Design review of the part built by this model. Coordinates are the model's own, in mm. Face numbers are marked on the shaded views. Give positions to 0.01 mm unless a question says otherwise; leave off trailing zeros. Loops run counter-clockwise (first coordinate to the right, second up) from the corner with the lowest first, then second, coordinate; pieces in that order, holes last.
from build123d import *

# Parameters (mm, degrees)
SKETCH1_R           = 6.5
BOSS_EXTRUDE1_DEPTH = 4
SKETCH2_R           = 2.75
CUT_EXTRUDE1_DEPTH  = 7
SKETCH3_R           = 0.9
CUT_EXTRUDE2_DEPTH  = 7


with BuildPart() as part:
    # Sketch1 → Boss-Extrude1 (new body)
    with BuildSketch(Plane(origin=(0, 0, 0), x_dir=(0, 0, -1), z_dir=(1, 0, 0))):
        Circle(SKETCH1_R)
    extrude(amount=BOSS_EXTRUDE1_DEPTH)

    # Sketch2 → Cut-Extrude1 (cut)
    with BuildSketch(Plane(origin=(4, 0, 0), x_dir=(0, 0, -1), z_dir=(1, 0, 0))):
        Circle(SKETCH2_R)
    extrude(amount=-CUT_EXTRUDE1_DEPTH, mode=Mode.SUBTRACT)

    # Sketch3 → Cut-Extrude2 (cut)
    with BuildSketch(Plane.ZY):
        with Locations((-2.001020721, 3.230466851)):
            Circle(SKETCH3_R)
        with Locations((3.798176719, 0.117701352)):
            Circle(SKETCH3_R)
        with Locations((-1.797155999, -3.348168203)):
            Circle(SKETCH3_R)
    extrude(amount=-CUT_EXTRUDE2_DEPTH, mode=Mode.SUBTRACT)


solid = part.part
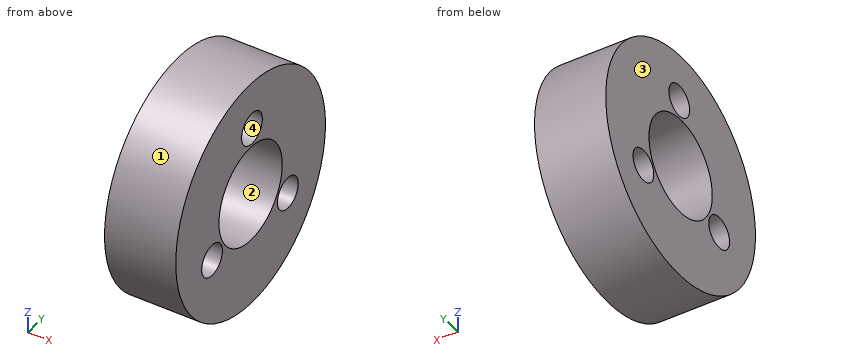
Q1. Take a section at B-B (y = 2.5). Give the boundary of the cut face in (x, z), plus the area to 3 significant figures.
Results:
outline: (0, -6) - (4, -6) - (4, -2.53) - (0, -2.53) - close; (0, -1.48) - (4, -1.48) - (4, -1.15) - (0, -1.15) - close; (0, 1.15) - (4, 1.15) - (4, 6) - (0, 6) - close
area: 34.6 mm2
Q2. Take a section at D-D (x = 0.4). Give the boundary of the cut face in (y, z).
Results:
outline: circle Ø13 at (0, 0); hole circle Ø1.8 at (-3.35, -1.8); hole circle Ø5.5 at (0, 0); hole circle Ø1.8 at (0.12, 3.8); hole circle Ø1.8 at (3.23, -2)
Q3. Take a section at C-C (z = -1.75). Give the boundary of the cut face in (x, y), plus the area to 3 significant figures.
Results:
outline: (0, -6.26) - (4, -6.26) - (4, -4.25) - (0, -4.25) - close; (0, -2.45) - (4, -2.45) - (4, -2.12) - (0, -2.12) - close; (0, 2.12) - (4, 2.12) - (4, 2.37) - (0, 2.37) - close; (0, 4.09) - (4, 4.09) - (4, 6.26) - (0, 6.26) - close
area: 19.0 mm2
Q4. Take a section at A-A (z = 0). Give the boundary of the cut face in (x, y).
Results:
outline: (0, -6.5) - (4, -6.5) - (4, -2.75) - (0, -2.75) - close; (0, 2.75) - (4, 2.75) - (4, 6.5) - (0, 6.5) - close
Q5. Wall thickness on line 1 (Z direction, x = 3.4, y = 2.5); line 2 (Z direction, x = 1, y = -0.5); line 3 (Y direction, x = 0.4, z = -2.25): over which ranges is each line inside the solid? List them lowest first.
Results:
line 1: z = -6 to -2.53, -1.48 to -1.15, 1.15 to 6
line 2: z = -6.48 to -2.7, 2.7 to 3.14, 4.45 to 6.48
line 3: y = -6.1 to -4.13, -2.57 to -1.58, 1.58 to 2.37, 4.1 to 6.1
Q6. Insertion check: pin 1 (1 mm diameter, centred on x = 3, z = -1.5, fed in from -Y); pin 2 (1.5 mm diameter, centred on x = 1.5, y = 1, fed in from -Z); pin 3 (1 mm diameter, centred on x = 2.5, y = 3, fed in from -Z). Each pin has a flat end and moves straight along its axis. Give the tip position at first contact, or say it passes through.
Results:
pin 1: stops at y = -6.42
pin 2: stops at z = -6.5
pin 3: stops at z = -6
Q7. Draft analysis for pull direction Y (two halves, no side actions). For the marked faces 1, 2, 3 and 4, state which applies: pulls with the +Y half, pulls with the -Y half, needs draft (parallel to the pull), parting line crosses it, or undercut.
Results:
face 1: parting line crosses it
face 2: undercut
face 3: needs draft
face 4: undercut
